```python
from build123d import *

# Parameters (mm, degrees)
SKETCH1_R           = 350
SKETCH1_R_2         = 200
BOSS_EXTRUDE1_DEPTH = 500
SKETCH2_R           = 100
BOSS_EXTRUDE2_DEPTH = 120
FILLET1_R           = 80
BOSS_EXTRUDE3_START = -60
BOSS_EXTRUDE3_DEPTH = 300
SKETCH4_R           = 75
CUT_EXTRUDE2_DEPTH  = 450


with BuildPart() as part:
    # Sketch1 → Boss-Extrude1 (new body)
    with BuildSketch(Plane.XY):
        Circle(SKETCH1_R)
        Circle(SKETCH1_R_2, mode=Mode.SUBTRACT)
    extrude(amount=BOSS_EXTRUDE1_DEPTH)

    # Sketch2 → Boss-Extrude2 (add)
    with BuildSketch(Plane.XY):
        with BuildLine():
            ThreePointArc((-141.421356237, -641.421356237), (0, -700), (141.421356237, -641.421356237))
            Line((141.421356237, -641.421356237), (641.421356237, -141.421356237))
            ThreePointArc((641.421356237, -141.421356237), (684.775906502, 76.536686473), (500, 200))
            Line((500, 200), (287.228132327, 200))
            ThreePointArc((287.228132327, 200), (333.938502059, 104.809717311), (350, 0))
            ThreePointArc((350, 0), (-104.809717311, -333.938502059), (-287.228132327, 200))
            Line((-287.228132327, 200), (-500, 200))
            ThreePointArc((-500, 200), (-684.775906502, 76.536686473), (-641.421356237, -141.421356237))
            Line((-641.421356237, -141.421356237), (-141.421356237, -641.421356237))
        make_face()
        with Locations((0, -500)):
            Circle(SKETCH2_R, mode=Mode.SUBTRACT)
        with Locations((-500, 0)):
            Circle(SKETCH2_R, mode=Mode.SUBTRACT)
        with Locations((500, 0)):
            Circle(SKETCH2_R, mode=Mode.SUBTRACT)
    extrude(amount=BOSS_EXTRUDE2_DEPTH)

    # Fillet1
    fillet1_edges = [part.edges().sort_by_distance(p)[0] for p in [
        (287.228132327, 200, 60),
        (-287.228132327, 200, 60),
    ]]
    fillet(fillet1_edges, radius=FILLET1_R)

    # Sketch3 → Boss-Extrude3 (add)
    with BuildSketch(Plane.XY.offset(500).offset(BOSS_EXTRUDE3_START)):
        with BuildLine():
            Line((225, 700), (125, 700))
            Line((125, 700), (125, 326.917420766))
            ThreePointArc((125, 326.917420766), (177.454262848, 301.678611434), (225, 268.095132369))
            Line((225, 268.095132369), (225, 700))
        make_face()
        with BuildLine():
            Line((-225, 700), (-225, 268.095132369))
            ThreePointArc((-225, 268.095132369), (-177.454262848, 301.678611434), (-125, 326.917420766))
            Line((-125, 326.917420766), (-125, 700))
            Line((-125, 700), (-225, 700))
        make_face()
    extrude(amount=-BOSS_EXTRUDE3_DEPTH)

    # Sketch4 → Cut-Extrude2 (cut)
    with BuildSketch(Plane(origin=(225, 0, 0), x_dir=(0, 0, -1), z_dir=(1, 0, 0))):
        with BuildLine():
            ThreePointArc((-440, 550), (-396.066017178, 656.066017178), (-290, 700))
            Line((-290, 700), (-440, 700))
            Line((-440, 700), (-440, 550))
        make_face()
        with BuildLine():
            ThreePointArc((-290, 700), (-183.933982822, 656.066017178), (-140, 550))
            Line((-140, 550), (-140, 700))
            Line((-140, 700), (-290, 700))
        make_face()
        with Locations((-290, 550)):
            Circle(SKETCH4_R)
    extrude(amount=-CUT_EXTRUDE2_DEPTH, mode=Mode.SUBTRACT)


solid = part.part
```
Geometry: final body of the model. Coordinates: model frame, mm. A direction names the side the tool comes from. Give positions to 0.01 mm unless a question says otherwise; leave off trailing zeros. Loops run counter-clockwise (first coordinate to the right, second up) from the corner with the lowest first, then second, coordinate; pieces in that order, holes last. Notation, with made-up numbers: (-12, -33) - (31, -33) arc R20 ccw to (31, -17) - close; hole circle Ø3 at (51, 20). An arc over 180 degrees is marked (long way). Answer as CSV lines item,"result". Start each with the question number.
(1) Mould query, pull axis Z, two halves, no side actions, for faces 4 (the face through (-3, -371, 120)), 5 (the face through (-174.3, 483.462, 255.392)), 6 (the face through (-225, 439, 292)). Classes: +Z half, -Z half, draft (parallel to the pull), parting line (faces both ways), or undercut.
(2) Section query A-A (x = 0). Output: boundary loops of the cut face in (y, z), and give its area (3 significant figures).
(3) Reachability of faces 1 (the face through (-412, 200, 59)), 2 (the face through (174, 411, 440)), 3 (the face through (174, 411, 140)) from +Z, -Z, +X, -X, +Y, -Y: full face, straight path, thin tool, end or side. Return the list, or none.
(4) Section query C-C (z = 348.5). Output: boundary loops of the cut face in (x, y), and give its area (3 significant figures).
(5) Section query B-B (y = 456.5). Output: boundary loops of the cut face in (x, z), and give its area (3 significant figures).
(6) Ray query, line 1 along Y through (x, z) = (0, 33); line 2 along Y through (x, z) = (0, 161); line 3 along Y through (x, z) = (166, 290). Return the intervals inside material, ascending. Write a range as [from, to].
(7) Pin query (flat end, axial travel): P1, Ø12, axis at y = -150.5, z = 362.5, coming from the -X side; P2, Ø1, axis at x = -195.5, z = 295.5, coming from the +Y side; P3, Ø12, axis at y = -105.5, z = 226, coming from the -X side. Return the tip coordinate at first contact, or that it passes through.
(8) Section query D-D (y = 75.5). Output: boundary loops of the cut face in (x, z), and give its area (3 significant figures).
Worked answers:
1,face 4,"+Z half"
1,face 5,"undercut"
1,face 6,"draft"
2,outline,"(-700, 0) - (-600, 0) - (-600, 120) - (-700, 120) - close; (-400, 0) - (-200, 0) - (-200, 500) - (-350, 500) - (-350, 120) - (-400, 120) - close; (200, 0) - (350, 0) - (350, 500) - (200, 500) - close"
2,area,"168,000 mm^2"
3,face 1,"+Z, -Z, -X, +Y"
3,face 2,"+Z, +X, +Y"
3,face 3,"-Z, +X, +Y"
4,outline,"(-225, 268.1) arc R350 ccw (long way) to (225, 268.1) - (225, 503.07) - (125, 503.07) - (125, 326.92) arc R350 ccw to (-125, 326.92) - (-125, 503.07) - (-225, 503.07) - close; (-225, 596.93) - (-125, 596.93) - (-125, 688.12) - (-225, 688.12) - close; (125, 596.93) - (225, 596.93) - (225, 688.12) - (125, 688.12) - close; hole circle Ø400 at (0, 0)"
4,area,"318,000 mm^2"
5,outline,"(-225, 140) - (-125, 140) - (-125, 440) - (-225, 440) - close; (125, 140) - (225, 140) - (225, 440) - (125, 440) - close"
5,area,"60,000 mm^2"
6,line 1,"y = [-700, -600], [-400, -200], [200, 350]"
6,line 2,"y = [-350, -200], [200, 350]"
6,line 3,"y = [-308.13, -111.55], [111.55, 475], [625, 700]"
7,P1,"stops at x = -318.78"
7,P2,"stops at y = 699.92"
7,P3,"stops at x = -335.56"
8,outline,"(-685.2, 0) - (-565.57, 0) - (-565.57, 120) - (-685.2, 120) - close; (-434.43, 0) - (-185.2, 0) - (-185.2, 500) - (-341.76, 500) - (-341.76, 120) - (-434.43, 120) - close; (185.2, 0) - (434.43, 0) - (434.43, 120) - (341.76, 120) - (341.76, 500) - (185.2, 500) - close; (565.57, 0) - (685.2, 0) - (685.2, 120) - (565.57, 120) - close"
8,area,"208,000 mm^2"
